Geometry: final body of the model. Coordinates: model frame, mm. Face numbers are marked on the shaded views. A direction names the side the tool comes from. Give positions to 0.01 mm unless a question says otherwise; leave off trailing zeros. Order: outer loops, then holes, each group sorted by start corner. A loop starts at its lowest first (then second) coordinate and runs counter-clockwise, first axis right, second up. Notation, with made-up numbers: (-2.75, 29.5) - (51.25, 29.5) arc R19 ccw to (51.25, 66.5) - close; hole circle Ø2 at (-2.75, -35.75). An arc over 180 degrees is marked (long way). Put each result on its own line as item: value. Start each with the question number.
1. Section C-C on x = 369. Return the cut outline in (y, z), plus the area to 3 significant figures.
2. Section A-A on y = 133. Return the cut outline in (x, z).
3. Section D-D on z = 449. Return the cut outline in (x, y), plus the area to 3 significant figures.
4. First-contact query: P1, Ø10, axis at x = 407.5, z = 219, coming from the +Y side; P2, Ø5, axis at x = 2, y = 509, coming from the -Z side; P3, Ø2, axis at y = 603.5, z = 247, coming from the -X side; P4, Ø1, axis at y = 35.5, z = 280.5, coming from the +X side. Flat tips, straight axial feed; report the tip coordinate or a pass-through.
5. Ray query, line 1 along X through (y, z) = (567, 233); line 2 along X through (y, z) = (617, 104.5); line 3 along Z through (x, y) = (564.5, 177). Return the intervals inside material, ascending. Write a range as from..to.
6. Mould query, pull axis Y, two halves, no side actions, for the marked faces 6, 7 and 8. Classes: pulls with the +Y half, pulls with the -Y half, needs draft (parallel to the pull), parting line crosses it, or undercut.
7. Set-up query: the marked faces 1, 2, 3, 4 and 5. Return all of +Z, -Z, +X, -X, +Y, -Y with unobstructed straight access to the full face (end or side cutting, diameter ignored); none if empty.
8. Section B-B on x = 71. Return the cut outline in (y, z), plus the area to 3 significant figures.
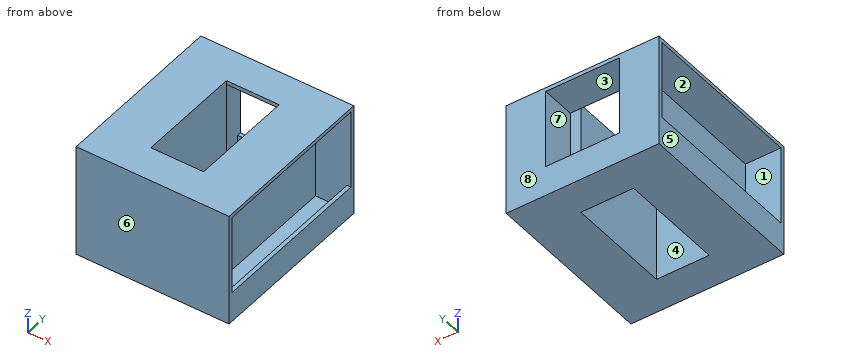
from build123d import *

# Parameters (mm, degrees)
F0_W      = 736.6
F0_H      = 838.2
F0_W_2    = 254
F0_H_2    = 508
F1_DEPTH  = 546.1
F2_W      = 800.1
F2_H      = 508
F3_DEPTH  = 171.45
F4_W      = 800.1
F4_H      = 508
F5_DEPTH  = 171.45
F6_W      = 19.05
F6_H      = 800.1
F7_DEPTH  = 127
F8_W      = 19.05
F8_H      = 800.1
F9_DEPTH  = 127
F10_W     = 355.6
F10_H     = 508
F11_DEPTH = 165.1
F12_W     = 355.6
F12_H     = 19.05
F13_DEPTH = 127


with BuildPart() as f1:
    # F0 (on Top) → F1 (new body)
    with BuildSketch(Plane.XY):
        with Locations((286.437001, 272.556877)):
            Rectangle(F0_W, F0_H)
        with Locations((286.437001, 272.556877)):
            Rectangle(F0_W_2, F0_H_2, mode=Mode.SUBTRACT)
    extrude(amount=F1_DEPTH)

    # F2 (on face) → F3 (cut)
    with BuildSketch(Plane.YZ.offset(654.737001)):
        with Locations((272.556877, 273.05)):
            Rectangle(F2_W, F2_H)
    extrude(amount=-F3_DEPTH, mode=Mode.SUBTRACT)

    # F4 (on face) → F5 (cut)
    with BuildSketch(Plane(origin=(-81.862999, 0, 0), x_dir=(0, -1, 0), z_dir=(-1, 0, 0))):
        with Locations((-272.556877, 273.05)):
            Rectangle(F4_W, F4_H)
    extrude(amount=-F5_DEPTH, mode=Mode.SUBTRACT)

    # F6 (on face) → F7 (join)
    with BuildSketch(Plane.XY.offset(19.05)):
        with Locations((645.212001, 272.556877)):
            Rectangle(F6_W, F6_H)
    extrude(amount=F7_DEPTH)

    # F8 (on face) → F9 (join)
    with BuildSketch(Plane.XY.offset(19.05)):
        with Locations((-72.337999, 272.556877)):
            Rectangle(F8_W, F8_H)
    extrude(amount=F9_DEPTH)

    # F10 (on face) → F11 (cut)
    with BuildSketch(Plane(origin=(0, 691.656877, 0), x_dir=(-1, 0, 0), z_dir=(0, 1, 0))):
        with Locations((-286.437001, 273.05)):
            Rectangle(F10_W, F10_H)
    extrude(amount=-F11_DEPTH, mode=Mode.SUBTRACT)

    # F12 (on face) → F13 (join)
    with BuildSketch(Plane.XY.offset(19.05)):
        with Locations((286.437001, 682.131877)):
            Rectangle(F12_W, F12_H)
    extrude(amount=F13_DEPTH)


solid = f1.part
Resolved:
1. outline: (-146.54, 0) - (18.56, 0) - (18.56, 546.1) - (-146.54, 546.1) - close; (526.56, 0) - (691.66, 0) - (691.66, 146.05) - (672.61, 146.05) - (672.61, 19.05) - (526.56, 19.05) - close; (526.56, 527.05) - (691.66, 527.05) - (691.66, 546.1) - (526.56, 546.1) - close
1. area: 98,900 mm^2
2. outline: (-81.86, 0) - (159.44, 0) - (159.44, 546.1) - (-81.86, 546.1) - (-81.86, 527.05) - (89.59, 527.05) - (89.59, 19.05) - (-62.81, 19.05) - (-62.81, 146.05) - (-81.86, 146.05) - close; (413.44, 0) - (654.74, 0) - (654.74, 146.05) - (635.69, 146.05) - (635.69, 19.05) - (483.29, 19.05) - (483.29, 527.05) - (654.74, 527.05) - (654.74, 546.1) - (413.44, 546.1) - close
3. outline: (-81.86, -146.54) - (654.74, -146.54) - (654.74, -127.49) - (483.29, -127.49) - (483.29, 672.61) - (654.74, 672.61) - (654.74, 691.66) - (464.24, 691.66) - (464.24, 526.56) - (413.44, 526.56) - (413.44, 18.56) - (159.44, 18.56) - (159.44, 526.56) - (108.64, 526.56) - (108.64, 691.66) - (-81.86, 691.66) - (-81.86, 672.61) - (89.59, 672.61) - (89.59, -127.49) - (-81.86, -127.49) - close
3. area: 155,000 mm^2
4. P1: y = 18.56
4. P2: z = 0
4. P3: x = 89.59
4. P4: x = 483.29
5. line 1: 89.59..108.64, 464.24..483.29
5. line 2: -81.86..-62.81, 89.59..108.64, 464.24..483.29, 635.69..654.74
5. line 3: 0..19.05, 527.05..546.1
6. face 6: pulls with the -Y half
6. face 7: undercut
6. face 8: pulls with the +Y half
7. face 1: none
7. face 2: -X
7. face 3: +Y
7. face 4: +Z, -Z
7. face 5: +Z, -Z, -X, +Y, -Y
8. outline: (-146.54, 0) - (691.66, 0) - (691.66, 546.1) - (-146.54, 546.1) - close; hole (-127.49, 19.05) - (672.61, 19.05) - (672.61, 527.05) - (-127.49, 527.05) - close
8. area: 51,300 mm^2
